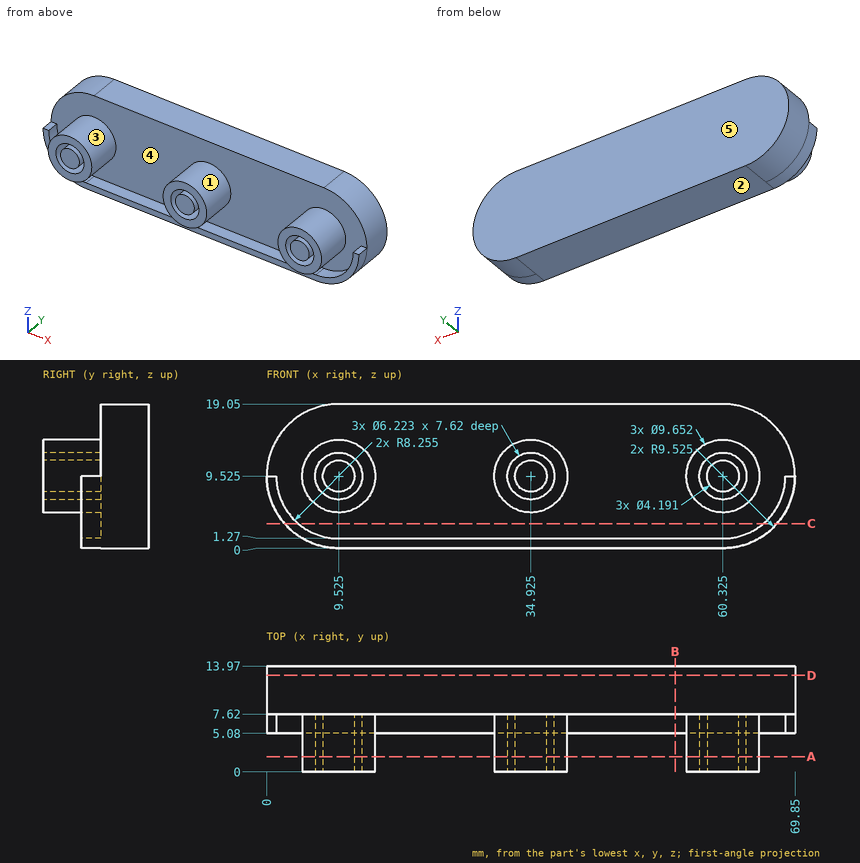
The drawing under review shows one solid part. Ordinate dimensions are in mm from its lowest x, y, z. A direction names the side the tool comes from. Coordinates: 2 decimals unless noted, no trailing zeros. Write each loop counter-clockwise with the first axis right and the second up, starting at its lowest first coordinate (ties: lowest second). Pieces come first, ordered by that corner, then holes.
1) Insertion check: pin 1 (2 mm diameter, centred on y = 5, z = 6.5, fed in from -X); pin 2 (6 mm diameter, centred on x = 47, z = 10, fed in from -Y); pin 3 (0.6 mm diameter, centred on x = 69, y = 6.5, fed in from +Z) (3 decimals). Each pin has a flat end and moves straight along its axis. Give the tip position at first contact, or say it passes through.
2) To check wall thickness, follow L1, parallel to X at y = 3.25, z = 13.75; L2, parallel to Y at x = 13, z = 1.5; L3, parallel to Z at x = 12, y = 2.5. State the ranges of each line that lie inside material, in increasing order.
3) Add section A-A (y = 2). State how many separate pieces and enclosed holes the cut face has, plus the area to 3 significant figures.
4) Add section D-D (y = 12.75). Write out the cut boundary in (x, z) (3 decimals).
5) Add section B-B (x = 54). Write out the cut boundary in (y, z), plus the area to 3 significant figures.
6) Add section C-C (z = 3.25). Write out the cut boundary in (x, y), plus the area to 3 significant figures.
7) Machinability: for the marked faces 1 and 2, which of the approach directions +Z, -Z, +X, -X, +Y, -Y give a long, thin tool a straight path to every point of the face, cutting with its end or side? Answer none if there is none.
8) Mouldability with a two-part tool opening along X and no side actions: class the marked faces 3, 4 and 5 as +X half, -X half, draft (parallel to the pull), parting line (faces both ways), or undercut.
Check result:
1. pin 1: stops at x = 0.22
1. pin 2: stops at y = 7.62
1. pin 3: stops at z = 9.525
2. L1: x = 7.19 to 11.86, 32.59 to 37.26, 57.99 to 62.66
2. L2: y = 7.62 to 13.97
2. L3: z = 5.38 to 7.64, 11.41 to 13.67
3. separate pieces: 6
3. enclosed holes: 3
3. area: 170 mm2
4. outline: (9.525, 0) - (60.325, 0) arc R9.525 ccw to (60.325, 19.05) - (9.525, 19.05) arc R9.525 ccw to start
5. outline: (5.08, 0) - (13.97, 0) - (13.97, 19.05) - (7.62, 19.05) - (7.62, 1.27) - (5.08, 1.27) - close
5. area: 124 mm2
6. outline: (2.36, 5.08) - (4.16, 5.08) - (4.16, 7.62) - (65.69, 7.62) - (65.69, 5.08) - (67.49, 5.08) - (67.49, 13.97) - (2.36, 13.97) - close
6. area: 423 mm2
7. face 1: -Y
7. face 2: -Z, +X, -X, +Y, -Y
8. face 3: undercut
8. face 4: undercut
8. face 5: draft
